Part model, mm, in its own coordinate system. A direction names the side the tool comes from. Give positions to 0.01 mm unless a question says otherwise; leave off trailing zeros. Order: outer loops, then holes, each group sorted by start corner. A loop starts at its lowest first (then second) coordinate and runs counter-clockwise, first axis right, second up. Notation, with made-up numbers: M 81,-30.75 L 131,-30.75 A21 cw 131,6.25 Z; hole C -25,43.5 d2. An arc over 180 degrees is marked long. Answer as a JSON object with one key per item and string values.
Autodesk Inventor part; units mm, degrees
ref_plane "YZ Plane" through (0, 0, 0) normal (1, 0, 0) x (0, 1, 0)
ref_plane "XZ Plane" through (0, 0, 0) normal (0, 1, 0) x (-1, 0, 0)
ref_plane "XY Plane" through (0, 0, 0) normal (0, 0, 1) x (1, 0, 0)
sketch "Skizze1" plane through (0, 0, 0) normal (0, 0, 1) x (1, 0, 0)
  line L0 (3, 3) -> (3, 25)
  line L1 (3, 25) -> (0, 25)
  line L2 (0, 25) -> (0, 0)
  line L3 (3, 3) -> (20, 3)
  line L4 (20, 3) -> (20, 0)
  line L5 (20, 0) -> (0, 0)
  dimension "d0" = 25
  dimension "d1" = 20
  dimension "d2" = 3
extrude "Extrusion1" add sketch "Skizze1" along normal blind 30
sketch "Skizze2" plane through (0, 0, 0) normal (0, -1, 0) x (1, 0, 0)
  line L0 (20, 30) -> (0, 30)
  line L1 (0, 0) -> (0, 30)
  line L2 (20, 0) -> (0, 0)
  line L3 (20, 0) -> (20, 30)
  line L4 (10, 30) -> (10, 0)
  line L5 (0, 15) -> (20, 15)
  point P0 (10, 25)
  point P1 (10, 5)
  dimension "d5" = 20
  dimension "d6" = 10
hole "Bohrung1" at (10, 0, 25) at (10, 0, 5) direction (0, 1, 0) diameter 4.5 end through all
sketch "Skizze3" plane through (3, 3, 0) normal (0, 1, 0) x (1, 0, 0)
  circle A0 centre (7, -25) radius 2.25
  line L0 (17, 0) -> (17, -30)
  line L1 (4, -22.75) -> (12, -22.75)
  line L2 (12, -27.25) -> (4, -27.25)
  arc A1 (4, -22.75) -> (4, -27.25) centre (4, -25) ccw
  arc A2 (12, -27.25) -> (12, -22.75) centre (12, -25) ccw
  point P0 (-3, 0)
  dimension "d14" = 5
  dimension "d15" = 8
extrude "Extrusion2" cut sketch "Skizze3" against normal through all contours A0 L1 A2 L2 | A0 L2 A1 L1
pattern_linear "Rechteckige Anordnung1" count 2 spacing 20 along (0, 0, -1) of "Extrusion2"
sketch "Skizze4" plane through (0, 0, 0) normal (-1, 0, 0) x (0, 0, 1)
  circle A0 centre (10, 17.5) radius 1.1
  circle A1 centre (19.4, 17.5) radius 1.1
hole "Bohrung2" at (0, 17.5, 10) at (0, 17.5, 19.4) direction (1, 0, 0) diameter 1.567 end through all
properties part number "13_0204_067"
1. Cut at C-C on y = 1.5. Give the cut face in (x, z).
Worked answers:
{"outline": "M 0,0 L 20,0 L 20,30 L 0,30 Z; hole M 7,2.75 L 15,2.75 A2.25 ccw 15,7.25 L 7,7.25 A2.25 ccw Z; hole M 7,22.75 L 15,22.75 A2.25 ccw 15,27.25 L 7,27.25 A2.25 ccw Z"}
2. Cut at D-D on y = 17.5. Give the cut face in (x, z).
Worked answers:
{"outline": "M 0,0 L 3,0 L 3,9.22 L 0,9.22 Z; M 0,10.78 L 3,10.78 L 3,18.62 L 0,18.62 Z; M 0,20.18 L 3,20.18 L 3,30 L 0,30 Z"}
3. Pin check, flat tips, straight feed: P1, Ø6, axis at x = 8, y = 17, coming from the +Z side; P2, Ø1, axis at y = 21, z = 14.5, coming from the +X side; P3, Ø4, axis at x = 11, z = 20, coming from the +Y side. Stop position of each tip, or through.
Worked answers:
{"P1": "passes through", "P2": "stops at x = 3", "P3": "stops at y = 3"}
4. Probe line 1 along Z through (x, y) = (0.8, 17.5); line 2 along Y through (x, z) = (1.6, 19.4); line 3 along X through (y, z) = (8.75, 21.75). List the from-to ranges inside material, lowest first.
Worked answers:
{"line 1": "z = 0 to 9.22, 10.78 to 18.62, 20.18 to 30", "line 2": "y = 0 to 16.72, 18.28 to 25", "line 3": "x = 0 to 3"}
5. Cut at B-B on z = 25. Give the cut face in (x, y), plus the area to 3 significant figures.
Worked answers:
{"outline": "M 0,0 L 4.75,0 L 4.75,3 L 3,3 L 3,25 L 0,25 Z; M 17.25,0 L 20,0 L 20,3 L 17.25,3 Z", "area": "88.5 mm^2"}
6. Two-plate mould, pull along Z, no slides. Class faces 1 (the flat face through (2.5, 8.9, 30)), 2 (the flat face through (11, 3, 15)), 3 (the flat face through (2.5, 8.9, 0)), 4 (the cylindrical face through (1.52, 16.84, 19.82)): +Z half, -Z half, draft (parallel to the pull), parting line (faces both ways), or undercut.
Worked answers:
{"face 1": "+Z half", "face 2": "draft", "face 3": "-Z half", "face 4": "undercut"}
7. Which spindle directions (+Z, -Z, +X, -X, +Y, -Y) get a long thin tool onto all of the face, cutting with end or side? Do faces 5 (the flat face through (11, 2, 7.25)), 6 (the flat face through (10, 0, 15)), 7 (the flat face through (3, 14, 15)). Say none if no direction does.
Worked answers:
{"face 5": "+Y, -Y", "face 6": "+Z, -Z, +X, -X, -Y", "face 7": "+Z, -Z, +X, +Y"}
8. Cut at A-A on x = 8.5. Give the cut face in (y, z), plus the area to 3 significant figures.
Worked answers:
{"outline": "M 0,0 L 3,0 L 3,2.75 L 0,2.75 Z; M 0,7.25 L 3,7.25 L 3,22.75 L 0,22.75 Z; M 0,27.25 L 3,27.25 L 3,30 L 0,30 Z", "area": "63.0 mm^2"}
